Geometry check sheet. Reference: the model listing, model coordinates, mm. Coordinates: 2 decimals unless noted, no trailing zeros. Write each loop counter-clockwise with the first axis right and the second up, starting at its lowest first coordinate (ties: lowest second). Pieces come first, ordered by that corner, then holes. Notation, with made-up numbers: M 4,61 L 23,61 A19 ccw 23,73 Z; hole C 48,20 d8. An arc over 180 degrees is marked long. Put each result on its own line as item: value. Start each with the question number.
1) Gauge pin test, flat ends, axial feed: pin 1 (1 mm diameter, centred on x = -138, z = 2, fed in from -Y); pin 2 (2.5 mm diameter, centred on x = 0, y = 100, fed in from -Z); pin 3 (1.5 mm diameter, centred on x = 17.5, z = 4, fed in from +Y); pin 4 (2 mm diameter, centred on x = 150, z = 2.5, fed in from -Y). Record the tip position at first contact, or that the pin passes through.
2) Cross-section at B-B on x = -142.5. Record the cut outline in (y, z), plus the area to 3 significant figures.
3) Mould release check, pull along X, two halves, no side actions. Record for faces 1 (the flat face through (-3, 3, 0)), 2 (the flat face through (92.621, 160.145, 2.535)), 3 (the cylindrical face through (-138.2, 137.57, 2.46)): released by +X, released by -X, zero draft, split by the parting line, or undercut.
4) Scan lines: line 1 along Y through (x, z) = (0, 3.8); line 2 along Y through (x, z) = (-100, 2.9). Record each from-to range of solid material in increasing order.
5) Cross-section at A-A on z = 2.3. Count the separate pieces of the cut face and the enclosed holes in it, plus the area to 3 significant figures.
6) Cross-section at C-C on y = 56.5. Record the cut outline in (x, z), plus the area to 3 significant figures.
Autodesk Inventor part; units mm, degrees
ref_plane "YZ Plane" through (0, 0, 0) normal (1, 0, 0) x (0, 1, 0)
ref_plane "XZ Plane" through (0, 0, 0) normal (0, 1, 0) x (-1, 0, 0)
ref_plane "XY Plane" through (0, 0, 0) normal (0, 0, 1) x (1, 0, 0)
sketch "Sketch1" plane through (0, 0, 0) normal (0, 0, 1) x (1, 0, 0)
  arc A0 (-19.0983, 194.0625) -> (19.0983, 194.0625) centre (0, 200) ccw
  arc A1 (-113.5709, 158.5139) -> (-80.4916, 177.6122) centre (-100, 173.2051) ccw
  arc A2 (-177.6122, 80.4916) -> (-158.5139, 113.5709) centre (-173.2051, 100) ccw
  arc A3 (-194.0625, -19.0983) -> (-194.0625, 19.0983) centre (-200, 0) ccw
  arc A4 (-158.5139, -113.5709) -> (-177.6122, -80.4916) centre (-173.2051, -100) ccw
  arc A5 (-80.4916, -177.6122) -> (-113.5709, -158.5139) centre (-100, -173.2051) ccw
  arc A6 (19.0983, -194.0625) -> (-19.0983, -194.0625) centre (0, -200) ccw
  arc A7 (113.5709, -158.5139) -> (80.4916, -177.6122) centre (100, -173.2051) ccw
  arc A8 (177.6122, -80.4916) -> (158.5139, -113.5709) centre (173.2051, -100) ccw
  arc A9 (194.0625, 19.0983) -> (194.0625, -19.0983) centre (200, 0) ccw
  arc A10 (158.5139, 113.5709) -> (177.6122, 80.4916) centre (173.2051, 100) ccw
  arc A11 (80.4916, 177.6122) -> (113.5709, 158.5139) centre (100, 173.2051) ccw
  arc A12 (-113.5709, 158.5139) -> (-158.5139, 113.5709) centre (0, 0) ccw
  arc A13 (-19.0983, 194.0625) -> (-80.4916, 177.6122) centre (0, 0) ccw
  arc A14 (158.5139, 113.5709) -> (19.0983, 194.0625) centre (0, 0) ccw
  arc A15 (194.0625, 19.0983) -> (177.6122, 80.4916) centre (0, 0) ccw
  arc A16 (177.6122, -80.4916) -> (194.0625, -19.0983) centre (0, 0) ccw
  arc A17 (19.0983, -194.0625) -> (158.5139, -113.5709) centre (0, 0) ccw
  arc A18 (-80.4916, -177.6122) -> (-19.0983, -194.0625) centre (0, 0) ccw
  arc A19 (-177.6122, 80.4916) -> (-177.6122, -80.4916) centre (0, 0) ccw
  arc A20 (-158.5139, -113.5709) -> (-113.5709, -158.5139) centre (0, 0) ccw
  line L0 (0, 0) -> (100, 0) construction
  circle A21 centre (-100, 0) radius 1.5
  circle A22 centre (0, -100) radius 1.5
  circle A23 centre (100, 0) radius 1.5
  circle A24 centre (0, 100) radius 1.5
  dimension "d4" = 40
  dimension "d5" = 360
  dimension "d9" = 3
  dimension "d12" = 360
extrude "Extrusion1" add sketch "Sketch1" along normal blind 5
sketch "Sketch2" plane through (0, 0, 5) normal (0, 0, 1) x (1, 0, 0)
  line L0 (0, 195) -> (10, 195)
  line L1 (10, 195) -> (10, 185)
  line L2 (10, 185) -> (0, 185)
  line L3 (0, 195) -> (-10, 195)
  line L4 (-10, 195) -> (-10, 185)
  line L5 (-10, 185) -> (0, 185)
  line L6 (-106.1603, 163.875) -> (-101.1603, 155.2147)
  line L7 (-97.5, 168.875) -> (-106.1603, 163.875)
  line L8 (-88.8397, 173.875) -> (-83.8397, 165.2147)
  line L9 (-97.5, 168.875) -> (-88.8397, 173.875)
  line L10 (-83.8397, 165.2147) -> (-92.5, 160.2147)
  line L11 (-101.1603, 155.2147) -> (-92.5, 160.2147)
  line L12 (-173.875, 88.8397) -> (-165.2147, 83.8397)
  line L13 (-168.875, 97.5) -> (-173.875, 88.8397)
  line L14 (-163.875, 106.1603) -> (-155.2147, 101.1603)
  line L15 (-168.875, 97.5) -> (-163.875, 106.1603)
  line L16 (-155.2147, 101.1603) -> (-160.2147, 92.5)
  line L17 (-165.2147, 83.8397) -> (-160.2147, 92.5)
  line L18 (-195, -10) -> (-185, -10)
  line L19 (-195, 0) -> (-195, -10)
  line L20 (-195, 10) -> (-185, 10)
  line L21 (-195, 0) -> (-195, 10)
  line L22 (-185, 10) -> (-185, 0)
  line L23 (-185, -10) -> (-185, 0)
  line L24 (-163.875, -106.1603) -> (-155.2147, -101.1603)
  line L25 (-168.875, -97.5) -> (-163.875, -106.1603)
  line L26 (-173.875, -88.8397) -> (-165.2147, -83.8397)
  line L27 (-168.875, -97.5) -> (-173.875, -88.8397)
  line L28 (-165.2147, -83.8397) -> (-160.2147, -92.5)
  line L29 (-155.2147, -101.1603) -> (-160.2147, -92.5)
  line L30 (-88.8397, -173.875) -> (-83.8397, -165.2147)
  line L31 (-97.5, -168.875) -> (-88.8397, -173.875)
  line L32 (-106.1603, -163.875) -> (-101.1603, -155.2147)
  line L33 (-97.5, -168.875) -> (-106.1603, -163.875)
  line L34 (-101.1603, -155.2147) -> (-92.5, -160.2147)
  line L35 (-83.8397, -165.2147) -> (-92.5, -160.2147)
  line L36 (10, -195) -> (10, -185)
  line L37 (0, -195) -> (10, -195)
  line L38 (-10, -195) -> (-10, -185)
  line L39 (0, -195) -> (-10, -195)
  line L40 (-10, -185) -> (0, -185)
  line L41 (10, -185) -> (0, -185)
  line L42 (106.1603, -163.875) -> (101.1603, -155.2147)
  line L43 (97.5, -168.875) -> (106.1603, -163.875)
  line L44 (88.8397, -173.875) -> (83.8397, -165.2147)
  line L45 (97.5, -168.875) -> (88.8397, -173.875)
  line L46 (83.8397, -165.2147) -> (92.5, -160.2147)
  line L47 (101.1603, -155.2147) -> (92.5, -160.2147)
  line L48 (173.875, -88.8397) -> (165.2147, -83.8397)
  line L49 (168.875, -97.5) -> (173.875, -88.8397)
  line L50 (163.875, -106.1603) -> (155.2147, -101.1603)
  line L51 (168.875, -97.5) -> (163.875, -106.1603)
  line L52 (155.2147, -101.1603) -> (160.2147, -92.5)
  line L53 (165.2147, -83.8397) -> (160.2147, -92.5)
  line L54 (195, 10) -> (185, 10)
  line L55 (195, 0) -> (195, 10)
  line L56 (195, -10) -> (185, -10)
  line L57 (195, 0) -> (195, -10)
  line L58 (185, -10) -> (185, 0)
  line L59 (185, 10) -> (185, 0)
  line L60 (163.875, 106.1603) -> (155.2147, 101.1603)
  line L61 (168.875, 97.5) -> (163.875, 106.1603)
  line L62 (173.875, 88.8397) -> (165.2147, 83.8397)
  line L63 (168.875, 97.5) -> (173.875, 88.8397)
  line L64 (165.2147, 83.8397) -> (160.2147, 92.5)
  line L65 (155.2147, 101.1603) -> (160.2147, 92.5)
  line L66 (88.8397, 173.875) -> (83.8397, 165.2147)
  line L67 (97.5, 168.875) -> (88.8397, 173.875)
  line L68 (106.1603, 163.875) -> (101.1603, 155.2147)
  line L69 (97.5, 168.875) -> (106.1603, 163.875)
  line L70 (101.1603, 155.2147) -> (92.5, 160.2147)
  line L71 (83.8397, 165.2147) -> (92.5, 160.2147)
  point P0 (0, 0)
  point P1 (0, 0)
  dimension "d16" = 10
  dimension "d17" = 10
  dimension "d20" = 360
extrude "Extrusion2" cut sketch "Sketch2" against normal blind 5 contours L19 L21 L20 L22 L23 L18 | L67 L69 L68 L70 L71 L66
properties part number "napduoinew"
Answer key:
1. pin 1: stops at y = -138.27
1. pin 2: passes through
1. pin 3: stops at y = 191.82
1. pin 4: stops at y = -125.79
2. outline: M -133.11,0 L 133.11,0 L 133.11,5 L -133.11,5 Z
2. area: 1,330 mm²
3. face 1: zero draft
3. face 2: undercut
3. face 3: released by -X
4. line 1: y = -180 to -101.5, -98.5 to 98.5, 101.5 to 180
4. line 2: y = -153.21 to -1.5, 1.5 to 153.21
5. separate pieces: 1
5. enclosed holes: 4
5. area: 115,000 mm²
6. outline: M -186.64,0 L 186.64,0 L 186.64,5 L -186.64,5 Z
6. area: 1,870 mm²
